Verification items for the finished model (mm, model axes). A direction names the side the tool comes from. Coordinates: 2 decimals unless noted, no trailing zeros. Write each loop counter-clockwise with the first axis right and the second up, starting at its lowest first coordinate (ties: lowest second). Pieces come first, ordered by that corner, then holes. Notation, with made-up numbers: (30.25, 42.5) -> (81.25, 42.5) arc R37 ccw to (81.25, 79.5) -> close; hole circle Ø8 at (5.5, 32.5). An arc over 180 degrees is marked (long way). Answer in a Markdown table with one row per item.
```python
from build123d import *

# Parameters (mm, degrees)
CYLINDER_R        = 28
CYLINDER_DEPTH    = 29
CYLINDER001_R     = 28
CYLINDER001_DEPTH = 29


with BuildPart() as cylinder:
    # Cylinder → Cylinder (new body)
    with BuildSketch(Plane(origin=(28, 0, 0), x_dir=(1, 0, 0), z_dir=(0, 0, 1))):
        Circle(CYLINDER_R)
    extrude(amount=CYLINDER_DEPTH)


with BuildPart() as sphere:
    # Sphere → Sphere (revolve)
    with BuildSketch(Plane(origin=(28, 0, 0), x_dir=(1, 0, 0), z_dir=(0, -1, 0))):
        with BuildLine():
            ThreePointArc((0, -28), (28, 0), (0, 28))
            Line((0, 28), (0, -28))
        make_face()
    revolve(axis=Axis((28, 0, 0), (0, 0, 1)))


with BuildPart() as fusion:
    # Cylinder001 → Cylinder001 (new body)
    with BuildSketch(Plane.ZY.offset(-28)):
        Circle(CYLINDER001_R)
    extrude(amount=CYLINDER001_DEPTH)

    # Fusion: union Cylinder, Sphere
    add(cylinder.part)
    add(sphere.part)


solid = fusion.part
```
1. Section check B-B, the plane z = -19. Record the boundary of the cut face in (x, y), plus the area to 3 significant figures.
Geometry says:
| item | result |
|---|---|
| outline | (-1, -20.57) -> (28, -20.57) arc R20.57 ccw to (28, 20.57) -> (-1, 20.57) -> close |
| area | 1,860 mm^2 |
2. Section check C-C, the plane x = 48. Record the boundary of the cut face in (y, z), plus the area to 3 significant figures.
Geometry says:
| item | result |
|---|---|
| outline | (-19.6, 0) arc R19.6 ccw to (19.6, 0) -> (19.6, 29) -> (-19.6, 29) -> close |
| area | 1,740 mm^2 |
3. Thickness scan on line 1 (Y direction, x = 18.5, z = 0); line 2 (X direction, y = 15.5, z = 15.5); line 3 (Z direction, x = 15, y = 7.5). Record the ranges inside material, lowest first. Write a range as from..to.
Geometry says:
| item | result |
|---|---|
| line 1 | -28..28 |
| line 2 | -1..51.32 |
| line 3 | -26.98..29 |
4. Section check D-D, the plane y = 15. Record the boundary of the cut face in (x, z).
Geometry says:
| item | result |
|---|---|
| outline | (-1, -23.64) -> (28, -23.64) arc R23.64 ccw to (51.64, 0) -> (51.64, 29) -> (4.36, 29) -> (4.36, 23.64) -> (-1, 23.64) -> close |
5. Section check A-A, the plane y = 0. Record the boundary of the cut face in (x, z).
Geometry says:
| item | result |
|---|---|
| outline | (-1, -28) -> (28, -28) arc R28 ccw to (56, 0) -> (56, 29) -> (0, 29) -> (0, 28) -> (-1, 28) -> close |
6. Depth check by flat-ended pin: P1, Ø1, axis at x = 7.5, z = 18.5, coming from the +Y side; P2, Ø1, axis at x = 5, z = 3.5, coming from the -Y side; P3, Ø8, axis at x = 31, y = 16, coming from the -Z side. Enter the tip coordinate at first touch or a pass-through.
Geometry says:
| item | result |
|---|---|
| P1 | y = 21.45 |
| P2 | y = -27.84 |
| P3 | z = -25.16 |
7. Tool access check on faces 1 (the flat face through (-1, 0, 0)), 2 (the cylindrical face through (54.707, 8.41, 14.297)), 3 (the cylindrical face through (13.703, 1.231, -27.973)). Record the directions out of +Z, -Z, +X, -X, +Y, -Y that give a thin tool (end or side, any length) a straight path to the whole face; none if there is none.
Geometry says:
| item | result |
|---|---|
| face 1 | +Z, -Z, -X, +Y, -Y |
| face 2 | +Z |
| face 3 | -X |
